Check sheet for the modelled part. Datum: model origin and axes. Units: mm. Round coordinates to 2 decimals unless told otherwise and drop trailing zeros. Order: outer loops, then holes, each group sorted by start corner. A loop starts at its lowest first (then second) coordinate and runs counter-clockwise, first axis right, second up. Notation, with made-up numbers: (-24.5, 2.25) -> (18.5, 2.25) arc R27 ccw to (18.5, 37.25) -> close; hole circle Ø3 at (82, 32). An arc over 180 degrees is marked (long way). Answer in a Markdown table with one row per item.
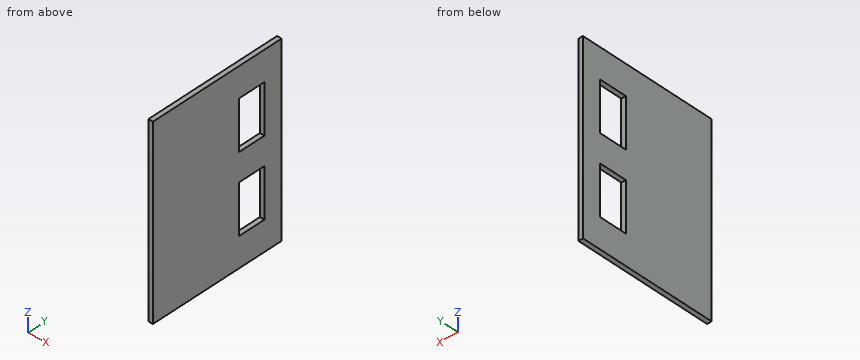
Autodesk Inventor part; units mm, degrees
ref_plane "YZ Plane" through (0, 0, 0) normal (1, 0, 0) x (0, 1, 0)
ref_plane "XZ Plane" through (0, 0, 0) normal (0, 1, 0) x (-1, 0, 0)
ref_plane "XY Plane" through (0, 0, 0) normal (0, 0, 1) x (1, 0, 0)
sketch "Sketch1" plane through (0, 0, 0) normal (0, 1, 0) x (-1, 0, 0)
  line L0 (-25, 1000) -> (25, 1000)
  line L1 (25, 1000) -> (25, -1000)
  line L2 (25, -1000) -> (-25, -1000)
  line L3 (-25, -1000) -> (-25, 1000)
  line L4 (-25, 1000) -> (25, -1000) construction
  line L5 (25, 1000) -> (-25, -1000) construction
  point P0 (0, 0)
  dimension "d0" = 50
  dimension "d1" = 2000
extrude "Extrusion1" add sketch "Sketch1" along normal blind 1500
sketch "Sketch2" plane through (25, 0, 1000) normal (1, 0, 0) x (0, 0, -1)
  line L0 (2000, 1500) -> (0, 1500)
  line L1 (1000, 1500) -> (1000, 0)
sketch "Sketch3" plane through (25, 0, 1000) normal (1, 0, 0) x (0, 0, -1)
  line L0 (1150, 1300) -> (1680, 1300)
  line L1 (1680, 1300) -> (1680, 1000)
  line L2 (1680, 1000) -> (1150, 1000)
  line L3 (1150, 1000) -> (1150, 1300)
  line L4 (2000, 0) -> (2000, 1500)
  line L5 (1000, 1500) -> (1000, 0)
  line L6 (0, 0) -> (2000, 0)
  dimension "d4" = 530
  dimension "d5" = 300
  dimension "d6" = 320
  dimension "d7" = 150
  dimension "d8" = 1000
extrude "Extrusion2" cut sketch "Sketch3" against normal through all
ref_plane "Work Plane1" through (-25, 0, 0) normal (0, 0, 1) x (1, 0, 0)
mirror "Mirror1" about plane through (-25, 0, 0) normal (0, 0, 1) of "Extrusion2"
properties part number "LCD PANEL"
Item 1: Scan lines: line 1 (Z direction, x = -21, y = 1231); line 2 (Y direction, x = -15, z = -580.5). Record each from-to range of solid material in increasing order. Write a range as [from, to].
Result sheet:
| item | result |
|---|---|
| line 1 | z = [-1000, -680], [-150, 150], [680, 1000] |
| line 2 | y = [0, 1000], [1300, 1500] |
Item 2: Cross-section at B-B (x = 4.5). Record the boundary of the cut face in (y, z).
Result sheet:
| item | result |
|---|---|
| outline | (0, -1000) -> (1500, -1000) -> (1500, 1000) -> (0, 1000) -> close; hole (1000, -680) -> (1300, -680) -> (1300, -150) -> (1000, -150) -> close; hole (1000, 150) -> (1300, 150) -> (1300, 680) -> (1000, 680) -> close |
Item 3: Cross-section at A-A (z = -534). Record the boundary of the cut face in (x, y), and give its area (3 significant figures).
Result sheet:
| item | result |
|---|---|
| outline | (-25, 0) -> (25, 0) -> (25, 1000) -> (-25, 1000) -> close; (-25, 1300) -> (25, 1300) -> (25, 1500) -> (-25, 1500) -> close |
| area | 60,000 mm^2 |
